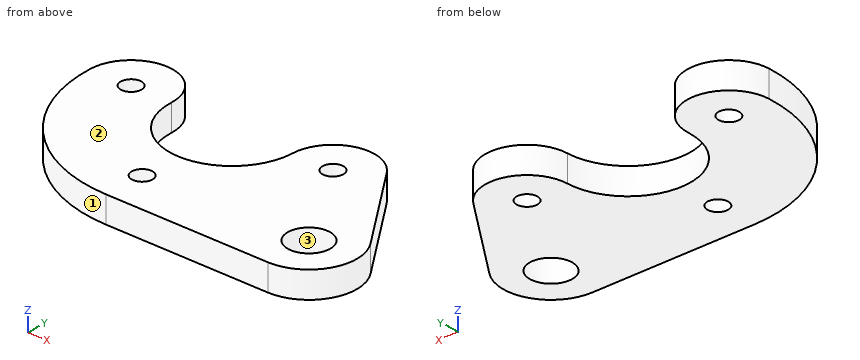
from build123d import *

# Parameters (mm, degrees)
SKETCH1_R           = 1.25
SKETCH1_R_2         = 2.5527
BOSS_EXTRUDE1_DEPTH = 3.175


with BuildPart() as part:
    # Sketch1 → Boss-Extrude1 (new body)
    with BuildSketch(Plane.XY):
        with BuildLine():
            Line((16.568712632, 2.906127581), (24.680172581, -8.450290414))
            ThreePointArc((24.680172581, -8.450290414), (25.11170139, -14.401205395), (20.017275273, -17.507075445))
            Line((20.017275273, -17.507075445), (-0.006184716, -17.499998907))
            ThreePointArc((-0.006184716, -17.499998907), (-12.376555105, -12.37218185), (-17.5, 0))
            ThreePointArc((-17.5, 0), (-12.5, 5), (-7.5, 0))
            ThreePointArc((-7.5, 0), (0, -7.5), (7.5, 0))
            ThreePointArc((7.5, 0), (10.974149935, 4.761489429), (16.568712632, 2.906127581))
        make_face()
        with Locations((12.5, 0)):
            Circle(SKETCH1_R, mode=Mode.SUBTRACT)
        with Locations((0, -12.5)):
            Circle(SKETCH1_R, mode=Mode.SUBTRACT)
        with Locations((-12.5, 0)):
            Circle(SKETCH1_R, mode=Mode.SUBTRACT)
        with Locations((20.019299513, -11.779375803)):
            Circle(SKETCH1_R_2, mode=Mode.SUBTRACT)
    extrude(amount=BOSS_EXTRUDE1_DEPTH)


solid = part.part
Design review of the part built by this model. Coordinates are the model's own, in mm. Face numbers are marked on the shaded views. Coordinates: 2 decimals unless noted, no trailing zeros. Order: outer loops, then holes, each group sorted by start corner. A loop starts at its lowest first (then second) coordinate and runs counter-clockwise, first axis right, second up. Notation, with made-up numbers: (-4.5, 66.25) -> (1.5, 66.25) arc R31 cw to (1.5, 100.25) -> close; hole circle Ø8 at (-20, 32). An arc over 180 degrees is marked (long way). One line per item, written item: value.
1) We need section D-D, the plane y = -16. Give the boundary of the cut face in (x, z) (3 decimals), then the cut area to 3 significant figures.
Output values:
outline: (-7.089, 0) -> (23.891, 0) -> (23.891, 3.175) -> (-7.089, 3.175) -> close
area: 98.4 mm2
2) To check wall thickness, follow probe 1 along Y at (x, z) = (12.5, 0.95); probe 2 along X at (y, z) = (1.75, 0.45); probe 3 along X at (y, z) = (4, 2.5). State the ranges of each line that lie inside material, in increasing order. Write a range as [from, to].
Output values:
probe 1: y = [-17.5, -1.25], [1.25, 5]
probe 2: x = [-17.18, -7.82], [7.82, 17.39]
probe 3: x = [-15.5, -9.5], [9.5, 15.5]
3) We need section A-A, the plane y = 3.5. Give the boundary of the cut face in (x, z) (3 decimals), then the cut area to 3 significant figures.
Output values:
outline: (-16.071, 0) -> (-8.929, 0) -> (-8.929, 3.175) -> (-16.071, 3.175) -> close; (8.929, 0) -> (16.071, 0) -> (16.071, 3.175) -> (8.929, 3.175) -> close
area: 45.3 mm2
4) Draft analysis for pull direction X (two halves, no side actions). For the marked faces 1, 2 and 3, state which applies: +X half, -X half, draft (parallel to the pull), parting line (faces both ways), or undercut.
Output values:
face 1: -X half
face 2: draft
face 3: undercut
5) We need section C-C, the plane z = 0.7. Give the boundary of the cut face in (x, y).
Output values:
outline: (-17.5, 0) arc R17.5 ccw to (-0.01, -17.5) -> (20.02, -17.51) arc R5.73 ccw to (24.68, -8.45) -> (16.57, 2.91) arc R5 ccw to (7.5, 0) arc R7.5 cw to (-7.5, 0) arc R5 ccw to start; hole circle Ø2.5 at (-12.5, 0); hole circle Ø2.5 at (0, -12.5); hole circle Ø2.5 at (12.5, 0); hole circle Ø5.11 at (20.02, -11.78)
6) We need section B-B, the plane x = 19. Give the boundary of the cut face in (y, z) (3 decimals), then the cut area to 3 significant figures.
Output values:
outline: (-17.507, 0) -> (-14.12, 0) -> (-14.12, 3.175) -> (-17.507, 3.175) -> close; (-9.439, 0) -> (-0.498, 0) -> (-0.498, 3.175) -> (-9.439, 3.175) -> close
area: 39.1 mm2
